```python
from build123d import *

# Parameters (mm, degrees)
SKETCH_1_R      = 1.25
PCB_DEPTH       = 1.5
SKETCH_6_W      = 5
SKETCH_6_H      = 5
EXTRUDE_2_DEPTH = 3
SKETCH_3_W      = 12
SKETCH_3_H      = 12
BUTTON_DEPTH    = 3
SKETCH_7_R      = 3.4
EXTRUDE_3_DEPTH = 7
FILLET_1_R      = 0.5


with BuildPart() as part:
    # 草图1 → 凸台-拉伸-PCB板 (new body)
    with BuildSketch(Plane(origin=(0, 0, 0), x_dir=(1, 0, 0), z_dir=(0, 1, 0))):
        with BuildLine():
            Line((-3, -8.5), (-3, -11.5))
            ThreePointArc((-3, -11.5), (0, -14.5), (3, -11.5))
            Line((3, -11.5), (3, -8.5))
            Line((3, -8.5), (6.5, -8.5))
            Line((6.5, -8.5), (6.5, 8.5))
            Line((6.5, 8.5), (3, 8.5))
            Line((3, 8.5), (3, 11.5))
            ThreePointArc((3, 11.5), (0, 14.5), (-3, 11.5))
            Line((-3, 11.5), (-3, 8.5))
            Line((-3, 8.5), (-6.5, 8.5))
            Line((-6.5, 8.5), (-6.5, -8.5))
            Line((-6.5, -8.5), (-3, -8.5))
        make_face()
        with Locations((0, -11.5)):
            Circle(SKETCH_1_R, mode=Mode.SUBTRACT)
        with Locations((0, 11.5)):
            Circle(SKETCH_1_R, mode=Mode.SUBTRACT)
    extrude(amount=PCB_DEPTH)

    # 草图6 → 凸台-拉伸2 (add)
    with BuildSketch(Plane.XZ):
        with Locations((2, 0)):
            Rectangle(SKETCH_6_W, SKETCH_6_H)
    extrude(amount=EXTRUDE_2_DEPTH)

    # 草图3 → 凸台-拉伸-Button-底座 (add)
    with BuildSketch(Plane(origin=(0, 1.5, 0), x_dir=(1, 0, 0), z_dir=(0, 1, 0))):
        Rectangle(SKETCH_3_W, SKETCH_3_H)
    extrude(amount=BUTTON_DEPTH)

    # 草图7 → 凸台-拉伸3 (add)
    with BuildSketch(Plane(origin=(0, 4.5, 0), x_dir=(1, 0, 0), z_dir=(0, 1, 0))):
        Circle(SKETCH_7_R)
    extrude(amount=EXTRUDE_3_DEPTH)

    # 圆角1
    fillet_1_edges = [part.edges().sort_by_distance(p)[0] for p in [
        (-3, 0.75, 8.5),
        (-6.5, 0.75, 8.5),
        (-6.5, 0.75, -8.5),
        (-3, 0.75, -8.5),
        (3, 0.75, -8.5),
        (6.5, 0.75, -8.5),
        (6.5, 0.75, 8.5),
        (3, 0.75, 8.5),
    ]]
    fillet(fillet_1_edges, radius=FILLET_1_R)


solid = part.part
```
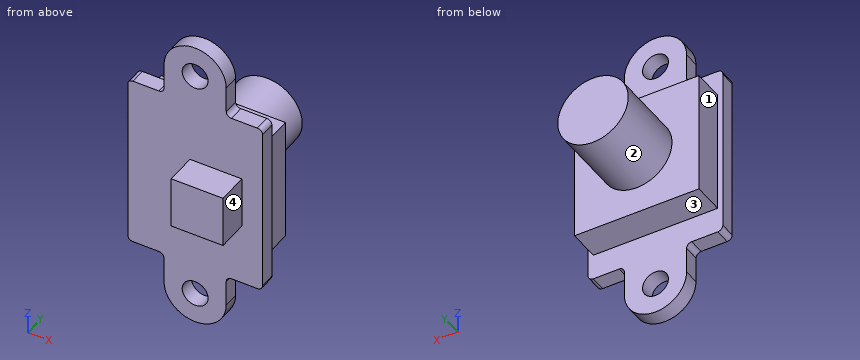
For this review, take the finished solid that the model builds, in its own axes (mm). Face numbers are marked on the shaded views. A direction names the side the tool comes from. Round coordinates to 2 decimals unless told otherwise and drop trailing zeros. Write each loop counter-clockwise with the first axis right and the second up, starting at its lowest first coordinate (ties: lowest second). Pieces come first, ordered by that corner, then holes.
1) Take a section at A-A on x = 0. Give the boundary of the cut face in (y, z).
Answer below:
outline: (-3, -2.5) - (0, -2.5) - (0, -10.25) - (1.5, -10.25) - (1.5, -6) - (4.5, -6) - (4.5, -3.4) - (11.5, -3.4) - (11.5, 3.4) - (4.5, 3.4) - (4.5, 6) - (1.5, 6) - (1.5, 10.25) - (0, 10.25) - (0, 2.5) - (-3, 2.5) - close; (0, -14.5) - (1.5, -14.5) - (1.5, -12.75) - (0, -12.75) - close; (0, 12.75) - (1.5, 12.75) - (1.5, 14.5) - (0, 14.5) - close
2) Take a section at C-C on x = -2.25. Give the boundary of the cut face in (y, z).
Answer below:
outline: (0, -13.48) - (1.5, -13.48) - (1.5, -6) - (4.5, -6) - (4.5, -2.55) - (11.5, -2.55) - (11.5, 2.55) - (4.5, 2.55) - (4.5, 6) - (1.5, 6) - (1.5, 13.48) - (0, 13.48) - close
3) Take a section at B-B on z = 0. Give the boundary of the cut face in (x, y).
Answer below:
outline: (-6.5, 0) - (-0.5, 0) - (-0.5, -3) - (4.5, -3) - (4.5, 0) - (6.5, 0) - (6.5, 1.5) - (6, 1.5) - (6, 4.5) - (3.4, 4.5) - (3.4, 11.5) - (-3.4, 11.5) - (-3.4, 4.5) - (-6, 4.5) - (-6, 1.5) - (-6.5, 1.5) - close
4) Take a section at D-D on y = 6.25. Give the boundary of the cut face in (x, z), then the cut area to 3 significant figures.
Answer below:
outline: circle Ø6.8 at (0, 0)
area: 36.3 mm2
5) Machinability: for the marked faces 1, 2, 3 and 4, which of the approach directions +Z, -Z, +X, -X, +Y, -Y give a long, thin tool a straight path to every point of the face, cutting with its end or side? Answer none if there is none.
Answer below:
face 1: +Z, -Z, -X, +Y
face 2: +Y
face 3: -Z, +X, -X, +Y
face 4: +Z, -Z, +X, -Y
6) For line 1 along X through (y, z) = (1.05, 11.5); line 2 along Z through (x, y) = (0, 0.5); line 3 along Y through (x, z) = (-3.25, 2), list the stretches that pass through material, from the lowest coordinate up.
Answer below:
line 1: x = -3 to -1.25, 1.25 to 3
line 2: z = -14.5 to -12.75, -10.25 to 10.25, 12.75 to 14.5
line 3: y = 0 to 4.5
7) Insertion check: pin 1 Ø1.2 at (y, z) = (0.5, 11) entering from +X; pin 2 Ø0.9 at (y, z) = (3, -2.5) entering from -X; pin 3 Ø0.8 at (x, y) = (-5, 1) entering from +Z; pin 4 Ø1.5 at (x, z) = (0, 11.5) entering from -Y. Each pin has a flat end and moves straight along its axis. Give the tip position at first contact, or say it passes through.
Answer below:
pin 1: stops at x = 3
pin 2: stops at x = -6
pin 3: stops at z = 8.5
pin 4: passes through
